Can you work these out from the model? Positions are in its coordinate system, mm. A direction names the side the tool comes from. Give positions to 0.01 mm unless a question says otherwise; leave off trailing zeros. Write each loop counter-clockwise with the first axis right and the second up, starting at its lowest first coordinate (ties: lowest second). Pieces come first, ordered by that corner, then holes.
from build123d import *

# Parameters (mm, degrees)
SKETCH1_R             = 40
SKETCH1_R_2           = 25
BOSS_EXTRUDE1_DEPTH   = 10
BOSS_EXTRUDE1_2_DEPTH = 10
BOSS_EXTRUDE1_3_DEPTH = 10
BOSS_EXTRUDE2_DEPTH   = 5


with BuildPart() as part:
    # Sketch1 → Boss-Extrude1 (new, symmetric)
    with BuildSketch(Plane(origin=(0, 0, 0), x_dir=(1, 0, 0), z_dir=(0, 1, 0))):
        with Locations(Location((0, -173.2, 0), (0, 0, 270))):
            Circle(SKETCH1_R)
        with Locations(Location((0, -173.2, 0), (0, 0, 270))):
            Circle(SKETCH1_R_2, mode=Mode.SUBTRACT)
    extrude(amount=BOSS_EXTRUDE1_DEPTH, both=True)



with BuildPart() as body_2:
    # Sketch1 → Boss-Extrude1 2 (new, symmetric)
    with BuildSketch(Plane(origin=(0, 0, 0), x_dir=(1, 0, 0), z_dir=(0, 1, 0))):
        with Locations(Location((-150, -86.6, 0), (0, 0, 270))):
            Circle(SKETCH1_R)
        with Locations(Location((-150, -86.6, 0), (0, 0, 270))):
            Circle(SKETCH1_R_2, mode=Mode.SUBTRACT)
    extrude(amount=BOSS_EXTRUDE1_2_DEPTH, both=True)


with BuildPart() as body_3:
    # Sketch1 → Boss-Extrude1 3 (new, symmetric)
    with BuildSketch(Plane(origin=(0, 0, 0), x_dir=(1, 0, 0), z_dir=(0, 1, 0))):
        with Locations(Location((0, 0, 0), (0, 0, 270))):
            Circle(SKETCH1_R)
        with Locations(Location((0, 0, 0), (0, 0, 270))):
            Circle(SKETCH1_R_2, mode=Mode.SUBTRACT)
    extrude(amount=BOSS_EXTRUDE1_3_DEPTH, both=True)


with BuildPart() as part_1:
    add(part.part)

    add(body_2.part)  # Boss-Extrude2 merges body 2

    add(body_3.part)  # Boss-Extrude2 merges body 3
    # Sketch1_3 → Boss-Extrude2 (add, symmetric)
    with BuildSketch(Plane(origin=(0, 0, 0), x_dir=(1, 0, 0), z_dir=(0, 1, 0))):
        with BuildLine():
            Line((10, -134.470166538), (10, -38.729833462))
            ThreePointArc((10, -38.729833462), (0, -40), (-10, -38.729833462))
            Line((-10, -38.729833462), (-10, -134.470166538))
            ThreePointArc((-10, -134.470166538), (0, -133.2), (10, -134.470166538))
        make_face()
        with BuildLine():
            ThreePointArc((-111.45884437, -97.304173145), (-115.358729812, -106.599559989), (-121.458624364, -114.624808239))
            Line((-121.458624364, -114.624808239), (-38.54115563, -162.495826855))
            ThreePointArc((-38.54115563, -162.495826855), (-34.641270188, -153.200440011), (-28.541375636, -145.175191761))
            Line((-28.541375636, -145.175191761), (-111.45884437, -97.304173145))
        make_face()
        with BuildLine():
            Line((-38.54115563, -10.704173145), (-121.458624364, -58.575191761))
            ThreePointArc((-121.458624364, -58.575191761), (-115.358729812, -66.600440011), (-111.45884437, -75.895826855))
            Line((-111.45884437, -75.895826855), (-28.541375636, -28.024808239))
            ThreePointArc((-28.541375636, -28.024808239), (-34.641270188, -19.999559989), (-38.54115563, -10.704173145))
        make_face()
    extrude(amount=BOSS_EXTRUDE2_DEPTH, both=True)


solid = part_1.part
(1) Imagine slicing it at B-B, the plane x = -150. Write out the boundary of the cut face in (y, z), plus the area to 3 significant figures.
Returned:
outline: (-10, 46.6) - (10, 46.6) - (10, 61.6) - (-10, 61.6) - close; (-10, 111.6) - (10, 111.6) - (10, 126.6) - (-10, 126.6) - close
area: 600 mm2
(2) Imagine slicing it at C-C, the plane y = -0.75. Write out the boundary of the cut face in (x, z).
Returned:
outline: (-121.46, 58.58) - (-38.54, 10.7) arc R40 ccw (long way) to (10, 38.73) - (10, 134.47) arc R40 ccw (long way) to (-38.54, 162.5) - (-121.46, 114.62) arc R40 ccw (long way) to start; hole circle Ø50 at (-150, 86.6); hole (-111.46, 75.9) - (-28.54, 28.02) arc R40 cw to (-10, 38.73) - (-10, 134.47) arc R40 cw to (-28.54, 145.18) - (-111.46, 97.3) arc R40 cw to start; hole circle Ø50 at (0, 0); hole circle Ø50 at (0, 173.2)
(3) If we mould it in two halves opening along X, with no side actions, what happens to faces 1 (the face through (7.509, -0.14, 23.846)), 2 (the face through (-75, -5, 130)), 3 (the face through (10, 0, 87))? For each: +X half, -X half, draft (parallel to the pull), parting line (faces both ways), or undercut.
Returned:
face 1: undercut
face 2: draft
face 3: +X half
(4) Imagine slicing it at D-D, the plane z = 173.2. Write out the boundary of the cut face in (x, y), plus the area to 3 significant figures.
Returned:
outline: (-40, -10) - (-25, -10) - (-25, 10) - (-40, 10) - close; (25, -10) - (40, -10) - (40, 10) - (25, 10) - close
area: 600 mm2
(5) Imagine slicing it at A-A, the plane z = 86.6. Write out the boundary of the cut face in (x, y), plus the area to 3 significant figures.
Returned:
outline: (-190, -10) - (-175, -10) - (-175, 10) - (-190, 10) - close; (-125, -10) - (-110, -10) - (-110, 10) - (-125, 10) - close; (-10, -5) - (10, -5) - (10, 5) - (-10, 5) - close
area: 800 mm2
(6) Will these pins go through, and if not, where does the flat tip stop? P1, Ø6, axis at x = -83, y = -1, coming from the +Z side; P2, Ø1, axis at y = -0.5, z = 94, coming from the -X side; P3, Ø5, axis at y = -2, z = 92, coming from the +X side.
Returned:
P1: stops at z = 138.56
P2: stops at x = -189.4
P3: stops at x = 10
(7) For faces 4 (the face through (-69.42, -0.07, 121.575)), 5 (the face through (18.34, -10, 17.22)), which set-ups out of +Z, -Z, +X, -X, +Y, -Y let a thin tool reach every point of the face, with its end or its side?
Returned:
face 4: +Y, -Y
face 5: +Z, -Z, +X, -X, -Y
(8) If I drill on L1, parallel to X at y = 0.5, z = 86.6; L2, parallel to X at y = -5.5, z = 0; L3, parallel to X at y = -7, z = 88.5, over which ranges is the centre line in solid material (lowest first)?
Returned:
L1: x = -190 to -175, -125 to -110, -10 to 10
L2: x = -40 to -25, 25 to 40
L3: x = -189.95 to -174.93, -125.07 to -110.05
